Can you work these out from the drawing? Everything is in mm from the part's minimum corner. A direction names the side the tool comes from. Coordinates: 2 decimals unless noted, no trailing zeros. Write each loop counter-clockwise with the first axis right and the second up, starting at its lowest first coordinate (ties: lowest second). Pieces come first, ordered by that corner, then holes. Notation, with made-up numbers: (-23.5, 35.25) -> (30.5, 35.25) arc R27 ccw to (30.5, 59.25) -> close; hole circle Ø1 at (-12.5, 2.25). An arc over 180 degrees is marked (long way). Use a Markdown table: item, result. Add a question column.
Item 1: If I drill on line 1 along Z through (x, y) = (67.5, 13.75); line 2 along Z through (x, y) = (14, 5); line 3 along X through (y, z) = (3, 22), over which ranges is the centre line in solid material (lowest first)? Write a range as from..to.
Item 2: Imagine slicing it at C-C, the plane z = 24.5. Write out the boundary of the cut face in (x, y), and give its area (3 significant figures).
Item 3: Imagine slicing it at A-A, the plane y = 5.25. Write out the boundary of the cut face in (x, z).
Item 4: Will these pins go through, and if not, where does the flat tip stop? pin 1 Ø4 at (x, z) = (32, 17) entering from -Y; pin 2 Ø5 at (y, z) = (12.5, 53.5) entering from +X; pin 3 Ø3 at (x, z) = (52, 53) entering from +Y.
Item 5: If we mould it in two halves opening along X, with no side actions, what happens to the marked faces 1, 2, 3 and 4? For each: pulls with the +X half, pulls with the -X half, needs draft (parallel to the pull), parting line crosses it, or undercut.
Item 6: Imagine slicing it at D-D, the plane y = 15.75. Write out the boundary of the cut face in (x, z).
Item 7: On a 3-axis mill with a long thin cutter (end or side, diameter ignored), from which of +Z, -Z, +X, -X, +Y, -Y can I reach the whole of each face in a straight line? I mean the marked faces 5, 6 and 7. Say none if no direction works.
Item 8: Imagine slicing it at B-B, the plane x = 62. Write out the boundary of the cut face in (y, z).
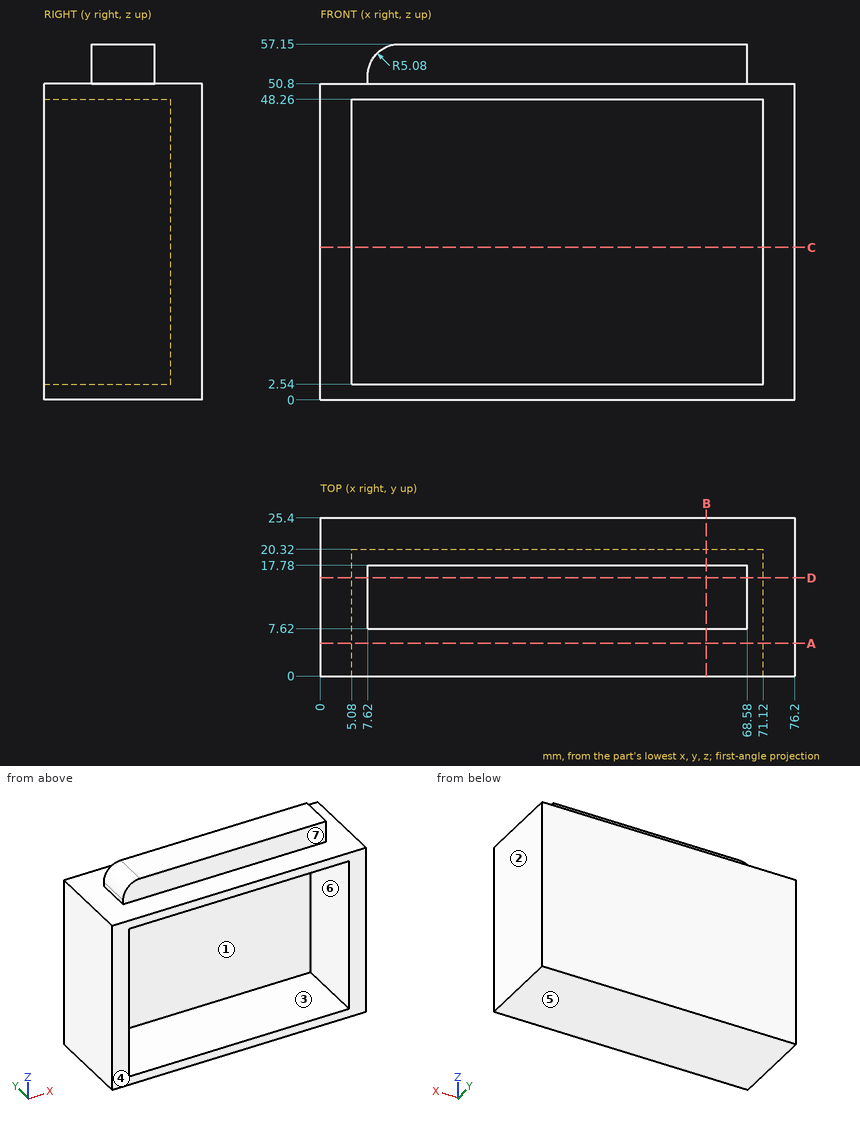
Ans:
| question | item | result |
|---|---|---|
| 1 | line 1 | z = 0..2.54, 48.26..57.15 |
| 1 | line 2 | z = 0..2.54, 48.26..50.8 |
| 1 | line 3 | x = 0..5.08, 71.12..76.2 |
| 2 | outline | (0, 0) -> (5.08, 0) -> (5.08, 20.32) -> (71.12, 20.32) -> (71.12, 0) -> (76.2, 0) -> (76.2, 25.4) -> (0, 25.4) -> close |
| 2 | area | 594 mm^2 |
| 3 | outline | (0, 0) -> (76.2, 0) -> (76.2, 50.8) -> (0, 50.8) -> close; hole (5.08, 2.54) -> (71.12, 2.54) -> (71.12, 48.26) -> (5.08, 48.26) -> close |
| 4 | pin 1 | stops at y = 20.32 |
| 4 | pin 2 | stops at x = 68.58 |
| 4 | pin 3 | stops at y = 17.78 |
| 5 | face 1 | undercut |
| 5 | face 2 | pulls with the +X half |
| 5 | face 3 | undercut |
| 5 | face 4 | needs draft |
| 6 | outline | (0, 0) -> (76.2, 0) -> (76.2, 50.8) -> (68.58, 50.8) -> (68.58, 57.15) -> (12.7, 57.15) arc R5.08 ccw to (7.62, 52.07) -> (7.62, 50.8) -> (0, 50.8) -> close; hole (5.08, 2.54) -> (71.12, 2.54) -> (71.12, 48.26) -> (5.08, 48.26) -> close |
| 7 | face 5 | -Z, +X, -X, +Y, -Y |
| 7 | face 6 | -Y |
| 7 | face 7 | +Z, +X, -X, -Y |
| 8 | outline | (0, 0) -> (25.4, 0) -> (25.4, 50.8) -> (17.78, 50.8) -> (17.78, 57.15) -> (7.62, 57.15) -> (7.62, 50.8) -> (0, 50.8) -> (0, 48.26) -> (20.32, 48.26) -> (20.32, 2.54) -> (0, 2.54) -> close |
